Geometry: see drawing. Coordinates: mm, zero at the bounding-box minimum. A direction names the side the tool comes from. Round coordinates to 2 decimals unless told otherwise and drop trailing zeros. Order: outer loops, then holes, each group sorted by start corner. A loop starts at its lowest first (then second) coordinate and runs counter-clockwise, first axis right, second up. Notation, with made-up numbers: (77.5, 12) - (95.5, 12) arc R18 cw to (95.5, 27) - close; hole circle Ø1 at (6, 19). An arc over 180 degrees is marked (long way). Put each result on its own line as item: value. Start each with the question number.
1) Line query: probe 1 along Z at (x, y) = (43, 214.5); probe 2 along Y at (x, z) = (20, 178.5); probe 3 along X at (y, z) = (69.5, 393). Output: solid intervals per line, ascending. Write a range as [from, to].
2) Section D-D on x = 146. Output: boundary loops of the cut face in (y, z).
3) Section B-B on y = 347.5. Output: boundary loops of the cut face in (x, z).
4) Section C-C on z = 371. Output: boundary loops of the cut face in (x, y).
5) Mould query, pull axis Y, two halves, no side actions, for the marked faces 3, 4 and 5. Classes: +Y half, -Y half, draft (parallel to the pull), parting line (faces both ways), or undercut.
6) Contact query for flat-ended pins moving along their axis: P1, Ø20, axis at x = 356, z = 39.5, coming from the -Y side; P2, Ø5, axis at y = 241.5, z = 243.5, coming from the -X side; P3, Ø6, axis at x = 255, y = 168.5, coming from the -Z side. Output: stop coordinate, or through.
7) Section A-A on x = 33.5. Output: boundary loops of the cut face in (y, z).
8) Access query for the marked faces 1 and 2. Directions: +Z, -Z, +X, -X, +Y, -Y. A direction counts if a zero-diameter tool reaches every point of the face in a straight line with its end or side. Return the directions, or none.
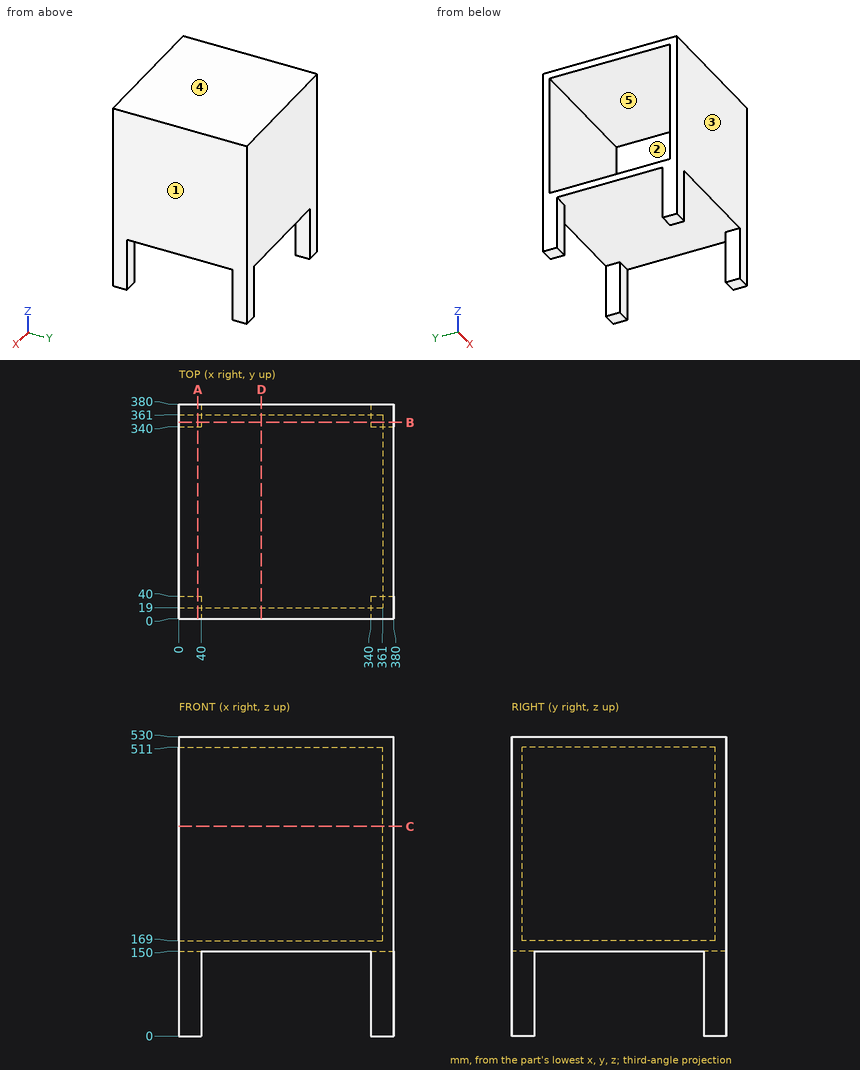
Answer sheet:
1. probe 1: [150, 169], [511, 530]
1. probe 2: [0, 19], [361, 380]
1. probe 3: [361, 380]
2. outline: (0, 150) - (380, 150) - (380, 530) - (0, 530) - close; hole (19, 169) - (361, 169) - (361, 511) - (19, 511) - close
3. outline: (0, 0) - (40, 0) - (40, 150) - (340, 150) - (340, 0) - (380, 0) - (380, 530) - (0, 530) - (0, 511) - (361, 511) - (361, 169) - (0, 169) - close
4. outline: (0, 0) - (380, 0) - (380, 380) - (0, 380) - (0, 361) - (361, 361) - (361, 19) - (0, 19) - close
5. face 3: -Y half
5. face 4: draft
5. face 5: undercut
6. P1: y = 0
6. P2: x = 361
6. P3: z = 150
7. outline: (0, 0) - (40, 0) - (40, 150) - (340, 150) - (340, 0) - (380, 0) - (380, 530) - (0, 530) - close; hole (19, 169) - (361, 169) - (361, 511) - (19, 511) - close
8. face 1: +Z, -Z, +X, +Y, -Y
8. face 2: -X
